Input: dimensioned drawing with shaded views. Units: mm. Origin: part minimum x, y, z. Give positions to 0.01 mm unless a question says otherwise; leave off trailing zeros. Order: outer loops, then holes, each group sorted by start corner. A loop starts at its lowest first (then second) coordinate and runs counter-clockwise, first axis right, second up. Notation, with made-up numbers: M -7,20 L 15,20 A20 cw 15,39 Z; hole C 58,50 d4. An arc over 180 degrees is marked long. Answer in a Markdown table with one row per item. Add a question column.
(1) Mould query, pull axis X, two halves, no side actions, for the marked faces 1 and 2. Classes: pulls with the +X half, pulls with the -X half, needs draft (parallel to the pull), parting line crosses it, or undercut.
(2) Section query D-D, the plane y = 24. Return loops of the section in (x, z), plus the area to 3 significant figures.
(3) Section query A-A, the plane x = 47.4. Return loops of the section in (y, z).
(4) Section query B-B, the plane y = 6.8. Return loops of the section in (x, z), plus the area to 3 significant figures.
(5) Material intervals for line 1 along Y through (x, z) = (47.4, 0.5); line 2 along Y through (x, z) = (3.2, 2.2); line 3 along Y through (x, z) = (9.5, 2), sorted ascending.
(6) Pin query (flat end, axial travel): P1, Ø6, axis at x = 37.5, y = 18.5, coming from the +Z side. Return the tip coordinate at first contact, or that it passes through.
(7) Section query C-C, the plane x = 40.5. Return loops of the section in (y, z).
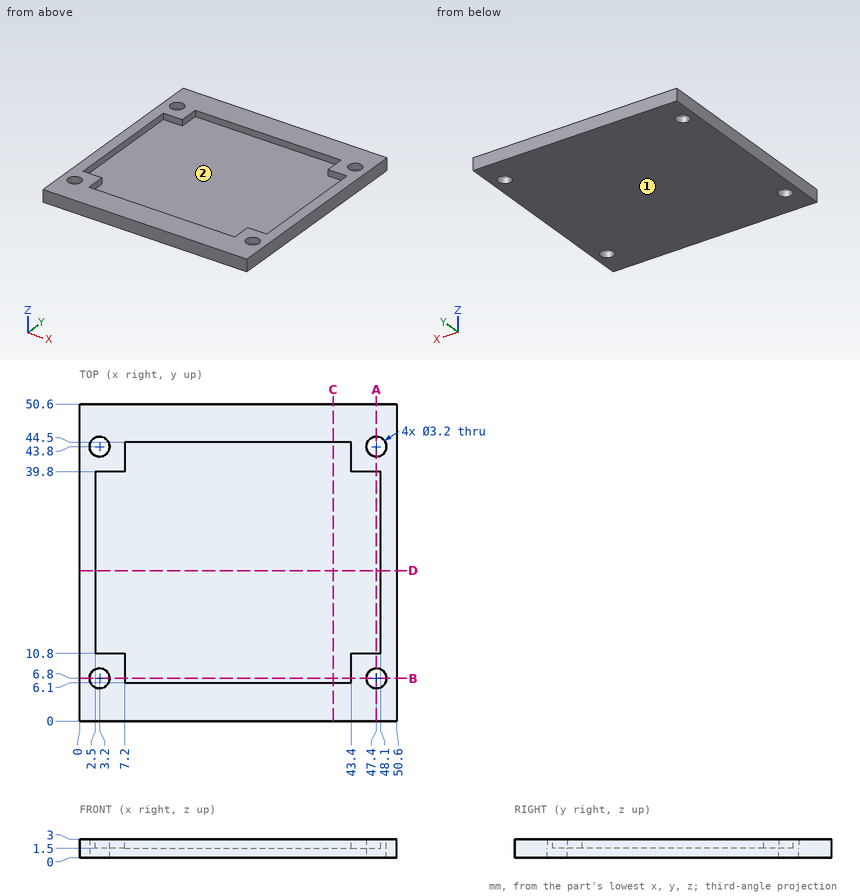
Values follow:
| question | item | result |
|---|---|---|
| 1 | face 1 | needs draft |
| 1 | face 2 | undercut |
| 2 | outline | M 0,0 L 50.6,0 L 50.6,3 L 48.1,3 L 48.1,1.5 L 2.5,1.5 L 2.5,3 L 0,3 Z |
| 2 | area | 83.4 mm² |
| 3 | outline | M 0,0 L 5.2,0 L 5.2,3 L 0,3 Z; M 8.4,0 L 42.2,0 L 42.2,3 L 39.8,3 L 39.8,1.5 L 10.8,1.5 L 10.8,3 L 8.4,3 Z; M 45.4,0 L 50.6,0 L 50.6,3 L 45.4,3 Z |
| 4 | outline | M 0,0 L 1.6,0 L 1.6,3 L 0,3 Z; M 4.8,0 L 45.8,0 L 45.8,3 L 43.4,3 L 43.4,1.5 L 7.2,1.5 L 7.2,3 L 4.8,3 Z; M 49,0 L 50.6,0 L 50.6,3 L 49,3 Z |
| 4 | area | 78.3 mm² |
| 5 | line 1 | y = 0 to 5.2, 8.4 to 42.2, 45.4 to 50.6 |
| 5 | line 2 | y = 0 to 5.2, 8.4 to 10.8, 39.8 to 42.2, 45.4 to 50.6 |
| 5 | line 3 | y = 0 to 6.1, 44.5 to 50.6 |
| 6 | P1 | stops at z = 1.5 |
| 7 | outline | M 0,0 L 50.6,0 L 50.6,3 L 44.5,3 L 44.5,1.5 L 6.1,1.5 L 6.1,3 L 0,3 Z |
